Geometry check sheet. Reference: the model listing, model coordinates, mm. Face numbers are marked on the shaded views. A direction names the side the tool comes from. Give positions to 0.01 mm unless a question says otherwise; leave off trailing zeros. Write each loop counter-clockwise with the first axis right and the second up, starting at its lowest first coordinate (ties: lowest second). Pieces come first, ordered by that corner, then holes. Notation, with made-up numbers: (78, 87.25) -> (134, 87.25) arc R15 cw to (134, 97.25) -> close; hole circle Ø1 at (-28, -17). An arc over 180 degrees is marked (long way). Write item = value, one per line. Start each with the question number.
1. Depth check by flat-ended pin: P1, Ø3, axis at y = 12, z = 4, coming from the +X side; P2, Ø3, axis at y = 1.5, z = 12, coming from the -X side; P3, Ø12, axis at x = 10, y = -2, coming from the +Z side; P4, Ø7, axis at x = -16, z = 7.05, coming from the +Y side. Enter the tip coordinate at first touch or a pass-through.
2. Cross-section at D-D, the plane y = -19. Record the cut outline in (x, z), plus the area to 3 significant figures.
3. Cross-section at B-B, the plane x = -16. Record the cut outline in (y, z).
4. Cross-section at C-C, the plane z = 7.05. Record the cut outline in (x, y) (3 decimals).
5. Thickness scan on line 1 along X through (y, z) = (13, 8.75) (3 decimals); line 2 along Z through (x, y) = (-16, -20); line 3 along X through (y, z) = (-18, 5.75). Record the ranges inside material, lowest first.
6. Mould release check, pull along Y, two halves, no side actions. Record for the marked faces 4, 5 and 6: pulls with the +Y half, pulls with the -Y half, needs draft (parallel to the pull), parting line crosses it, or undercut.
7. Set-up check for the marked faces 1, 2 and 3: record each of +Z, -Z, +X, -X, +Y, -Y from which the full face is reachable in a straight line by a thin tool's end or side.
8. Cross-section at A-A, the plane y = 6.5. Record the cut outline in (x, z) (3 decimals).
```python
from build123d import *

# Parameters (mm, degrees)
F1_DEPTH = 14.1
F2_R     = 2.75
F3_DEPTH = 38.801
F4_SIZE  = 0.5


with BuildPart() as f1:
    # F0 (on Top) → F1 (new body)
    with BuildSketch(Plane.XY):
        with BuildLine():
            ThreePointArc((0.675, 4.81191), (0, -7.15), (-0.675, 4.81191))
            Line((-0.675, 4.81191), (-0.675, 15))
            Line((-0.675, 15), (-10, 15))
            Line((-10, 15), (-10, -17.3))
            Line((-10, -17.3), (-21, -17.3))
            Line((-21, -17.3), (-21, -23.8))
            Line((-21, -23.8), (21, -23.8))
            Line((21, -23.8), (21, -17.3))
            Line((21, -17.3), (10, -17.3))
            Line((10, -17.3), (10, 15))
            Line((10, 15), (0.675, 15))
            Line((0.675, 15), (0.675, 4.81191))
        make_face()
    extrude(amount=F1_DEPTH)

    # F2 (on face) → F3 (cut, through all)
    with BuildSketch(Plane.XZ.offset(23.8)):
        with Locations((16, 7.05)):
            Circle(F2_R)
        with Locations((-16, 7.05)):
            Circle(F2_R)
    extrude(amount=-F3_DEPTH, mode=Mode.SUBTRACT)

    # F4
    f4_edges = [f1.edges().sort_by_distance(p)[0] for p in [
        (10, -1.15, 14.1),
        (15.5, -17.3, 14.1),
        (21, -20.55, 14.1),
        (21, -17.3, 7.05),
        (21, -23.8, 7.05),
        (21, -20.55, 0),
        (0, -23.8, 14.1),
        (-15.5, -17.3, 14.1),
        (-21, -20.55, 14.1),
        (-10, -1.15, 14.1),
        (-5.3375, 15, 14.1),
        (5.3375, 15, 14.1),
        (0, -7.15, 14.1),
        (-21, -17.3, 7.05),
        (-21, -23.8, 7.05),
        (-21, -20.55, 0),
        (-15.5, -17.3, 0),
        (-10, -1.15, 0),
        (0, -23.8, 0),
        (0, -7.15, 0),
        (-10, 15, 7.05),
        (-5.3375, 15, 0),
        (5.3375, 15, 0),
        (10, -1.15, 0),
        (15.5, -17.3, 0),
        (10, 15, 7.05),
    ]]
    chamfer(f4_edges, length=F4_SIZE)


solid = f1.part
```
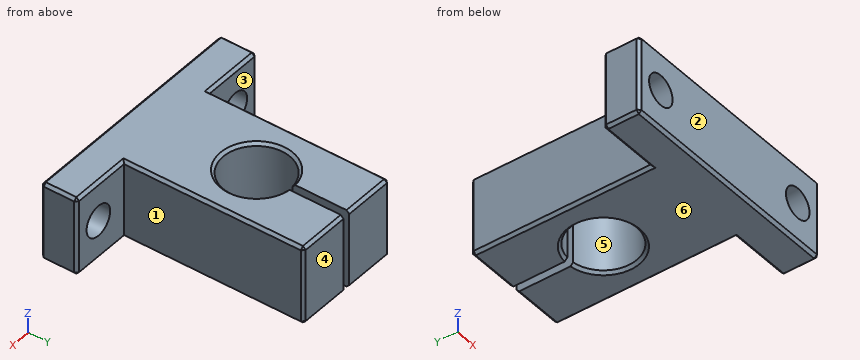
Answers:
q1.P1 = 10
q1.P2 = -10
q1.P3 = 14.1
q1.P4 = -17.3
q2.outline = (-21, 0.5) -> (-20.5, 0) -> (20.5, 0) -> (21, 0.5) -> (21, 13.6) -> (20.5, 14.1) -> (-20.5, 14.1) -> (-21, 13.6) -> close; hole circle Ø5.5 at (-16, 7.05); hole circle Ø5.5 at (16, 7.05)
q2.area = 544 mm^2
q3.outline = (-23.8, 0.5) -> (-23.3, 0) -> (-17.8, 0) -> (-17.3, 0.5) -> (-17.3, 4.3) -> (-23.8, 4.3) -> close; (-23.8, 9.8) -> (-17.3, 9.8) -> (-17.3, 13.6) -> (-17.8, 14.1) -> (-23.3, 14.1) -> (-23.8, 13.6) -> close
q4.outline = (-21, -23.3) -> (-20.5, -23.8) -> (-18.75, -23.8) -> (-18.75, -17.3) -> (-20.5, -17.3) -> (-21, -17.8) -> close; (-13.25, -23.8) -> (13.25, -23.8) -> (13.25, -17.3) -> (10, -17.3) -> (10, 14.5) -> (9.5, 15) -> (0.675, 15) -> (0.675, 4.812) arc R6 cw (long way) to (-0.675, 4.812) -> (-0.675, 15) -> (-9.5, 15) -> (-10, 14.5) -> (-10, -17.3) -> (-13.25, -17.3) -> close; (18.75, -23.8) -> (20.5, -23.8) -> (21, -23.3) -> (21, -17.8) -> (20.5, -17.3) -> (18.75, -17.3) -> close
q5.line_1 = -10 to -0.675, 0.675 to 10
q5.line_2 = 0 to 4.3, 9.8 to 14.1
q5.line_3 = -21 to -18.42, -13.58 to 13.58, 18.42 to 21
q6.face_4 = pulls with the +Y half
q6.face_5 = undercut
q6.face_6 = needs draft
q7.face_1 = +Z, -Z, +X, +Y
q7.face_2 = +Z, -Z, +X, -X, -Y
q7.face_3 = +Z, -Z, -X, +Y
q8.outline = (-10, 0.5) -> (-9.5, 0) -> (-0.675, 0) -> (-0.675, 14.1) -> (-9.5, 14.1) -> (-10, 13.6) -> close; (0.675, 0) -> (9.5, 0) -> (10, 0.5) -> (10, 13.6) -> (9.5, 14.1) -> (0.675, 14.1) -> close
